Model file for the job. Use its own axes, mm. A direction names the side the tool comes from. Round coordinates to 2 decimals unless told otherwise and drop trailing zeros. Order: outer loops, then holes, each group sorted by start corner. A loop starts at its lowest first (then second) coordinate and runs counter-clockwise, first axis right, second up. Notation, with made-up numbers: M -11,57.5 L -5,57.5 A27 ccw -5,96.5 Z; hole C 39,-16 d5. An arc over 180 degrees is marked long. Return JSON: item names as keys, results as strings. Group by question number.
Item 1: Slice it at A-A on z = 100. Write the cut outline in (x, y).
Item 2: Slice it at C-C on y = 35. Write the cut outline in (x, z), then the cut area to 3 significant figures.
Item 3: Pin check, flat tips, straight feed: pin 1 Ø8 at (y, z) = (68.5, -45) entering from -X; pin 2 Ø12 at (x, z) = (65, 105) entering from -Y; pin 3 Ø10 at (x, z) = (33, 48) entering from +Y; pin 4 Ø10.5 at (x, z) = (70, 100) entering from +Y. Stop position of each tip, or through.
Item 4: Slice it at D-D on z = -37.5. Write the cut outline in (x, y), then the cut area to 3 significant figures.
Item 5: Probe line 1 along Z through (x, y) = (70, 131); line 2 along Y through (x, z) = (15.5, 40); line 3 along X through (y, z) = (67, 87). List the from-to ranges inside material, lowest first.
Item 6: Slice it at B-B on x = 70. Write the cut outline in (y, z), then the cut area to 3 significant figures.
Item 7: Pull direction Y, two halves, no side cores. Call faces 4 (the face through (1, 133, 100)), 5 (the face through (-1, -129, 2)), 6 (the face through (-71.846, 131.479, 96.451)): pulls with the +Y half, pulls with the -Y half, needs draft (parallel to the pull), parting line crosses it, or undercut.
Item 8: Which spindle directions (+Z, -Z, +X, -X, +Y, -Y) get a long thin tool onto all of the face, cutting with end or side? Do faces 1 (the face through (-50, -2, 2)), 2 (the face through (-1, 130, 142)), 3 (the face through (50, -2, 2)). Say none if no direction does.
from build123d import *

# Parameters (mm, degrees)
F0_W     = 100
F0_H     = 260
F1_DEPTH = 165
F2_T     = -1
F4_DEPTH = 220
F5_R     = 1
F6_W     = 180
F6_H     = 40
F6_R     = 4
F7_DEPTH = 3


with BuildPart() as f1:
    # F0 (on Top) → F1 (new body, symmetric)
    with BuildSketch(Plane.XY):
        Rectangle(F0_W, F0_H)
    extrude(amount=F1_DEPTH, both=True)

    # F2 (hollow: no face is removed)
    offset(amount=F2_T, mode=Mode.SUBTRACT)

    # F3 (on face) → F4 (cut, symmetric)
    with BuildSketch(Plane.XZ.offset(130)):
        with BuildLine():
            Line((-18, -150), (-22, -150))
            ThreePointArc((-22, -150), (-24.1213203436, -150.8786796564), (-25, -153))
            Line((-25, -153), (-25, -157))
            ThreePointArc((-25, -157), (-24.1213203436, -159.1213203436), (-22, -160))
            Line((-22, -160), (22, -160))
            ThreePointArc((22, -160), (24.1213203436, -159.1213203436), (25, -157))
            Line((25, -157), (25, -153))
            ThreePointArc((25, -153), (24.1213203436, -150.8786796564), (22, -150))
            Line((22, -150), (18, -150))
            ThreePointArc((18, -150), (15.8786796564, -149.1213203436), (15, -147))
            Line((15, -147), (15, -143))
            ThreePointArc((15, -143), (14.1213203436, -140.8786796564), (12, -140))
            Line((12, -140), (-12, -140))
            ThreePointArc((-12, -140), (-14.1213203436, -140.8786796564), (-15, -143))
            Line((-15, -143), (-15, -147))
            ThreePointArc((-15, -147), (-15.8786796564, -149.1213203436), (-18, -150))
        make_face()
    extrude(amount=F4_DEPTH, both=True, mode=Mode.SUBTRACT)

    # F5
    f5_edges = [f1.edges().sort_by_distance(p)[0] for p in [
        (50, 0, -165),
        (50, 130, 0),
        (50, 0, 165),
        (50, -130, 0),
        (0, 130, 165),
        (-50, 0, 165),
        (0, -130, 165),
        (-50, 130, 0),
        (-50, 0, -165),
        (-50, -130, 0),
        (0, 130, -165),
        (0, -130, -165),
    ]]
    fillet(f5_edges, radius=F5_R)

    # F6 (on face) → F7 (join)
    with BuildSketch(Plane(origin=(0, 130, 0), x_dir=(-1, 0, 0), z_dir=(0, 1, 0))):
        with Locations((0, 100)):
            Rectangle(F6_W, F6_H)
        with Locations((-70, 100)):
            Circle(F6_R, mode=Mode.SUBTRACT)
        with Locations((70, 100)):
            Circle(F6_R, mode=Mode.SUBTRACT)
        with Locations((0, -100)):
            Rectangle(F6_W, F6_H)
        with Locations((-70, -100)):
            Circle(F6_R, mode=Mode.SUBTRACT)
        with Locations((70, -100)):
            Circle(F6_R, mode=Mode.SUBTRACT)
    extrude(amount=F7_DEPTH)


solid = f1.part
Output values:
{
 "1": {"outline": "M -90,130 L -74,130 L -74,133 L -90,133 Z; M -66,130 L -49,130 A1 ccw -50,129 L -50,-129 A1 ccw -49,-130 L 49,-130 A1 ccw 50,-129 L 50,129 A1 ccw 49,130 L 66,130 L 66,133 L -66,133 Z; M 74,130 L 90,130 L 90,133 L 74,133 Z; hole M -49,-129 L 49,-129 L 49,129 L -49,129 Z"},
 "2": {"outline": "M -50,-164 A1 ccw -49,-165 L 49,-165 A1 ccw 50,-164 L 50,164 A1 ccw 49,165 L -49,165 A1 ccw -50,164 Z; hole M -49,-164 L 49,-164 L 49,164 L -49,164 Z", "area": "855 mm²"},
 "3": {"pin 1": "x = -50", "pin 2": "y = 130", "pin 3": "y = 130", "pin 4": "y = 133"},
 "4": {"outline": "M -50,-129 A1 ccw -49,-130 L 49,-130 A1 ccw 50,-129 L 50,129 A1 ccw 49,130 L -49,130 A1 ccw -50,129 Z; hole M -49,-129 L 49,-129 L 49,129 L -49,129 Z", "area": "715 mm²"},
 "5": {"line 1": "-120 to -104, -96 to -80, 80 to 96, 104 to 120", "line 2": "-130 to -129, 129 to 130", "line 3": "-50 to -49, 49 to 50"},
 "6": {"outline": "M 130,-120 L 133,-120 L 133,-104 L 130,-104 Z; M 130,-96 L 133,-96 L 133,-80 L 130,-80 Z; M 130,80 L 133,80 L 133,96 L 130,96 Z; M 130,104 L 133,104 L 133,120 L 130,120 Z", "area": "192 mm²"},
 "7": {"face 4": "pulls with the +Y half", "face 5": "undercut", "face 6": "needs draft"},
 "8": {"face 1": "+Z, -Z, -X, -Y", "face 2": "+Z, +X, -X, +Y", "face 3": "+Z, -Z, +X, -Y"}
}
